```python
from build123d import *

# Parameters (mm, degrees)
F0_R     = 21.5
F1_DEPTH = 3
F2_R     = 1
F3_DEPTH = 3
F4_D     = 3


with BuildPart() as f1:
    # F0 (on Top) → F1 (new body)
    with BuildSketch(Plane.XY):
        Circle(F0_R)
    extrude(amount=F1_DEPTH)

    # F2 (on face) → F3 (join)
    with BuildSketch(Plane.XY.offset(3)):
        with BuildLine():
            Line((-1.347391, 11.193886), (0, 21.5))
            Line((0, 21.5), (-4.736634, 11.324242))
            Line((-4.736634, 11.324242), (-1.543514, 3.690199))
            ThreePointArc((-1.543514, 3.690199), (-3.859717, 1.050041), (-3.200264, -2.399647))
            Line((-3.200264, -2.399647), (-9.020494, -6.763818))
            Line((-9.020494, -6.763818), (-18.619546, -10.75))
            Line((-18.619546, -10.75), (-7.438764, -9.764166))
            Line((-7.438764, -9.764166), (-2.424049, -3.181821))
            ThreePointArc((-2.424049, -3.181821), (1.020496, -3.867633), (3.678288, -1.571687))
            Line((3.678288, -1.571687), (10.367886, -4.430068))
            Line((10.367886, -4.430068), (18.619546, -10.75))
            Line((18.619546, -10.75), (12.175398, -1.560076))
            Line((12.175398, -1.560076), (3.967563, -0.508377))
            ThreePointArc((3.967563, -0.508377), (2.839221, 2.817592), (-0.478023, 3.971334))
            Line((-0.478023, 3.971334), (-1.347391, 11.193886))
        make_face()
        Circle(F2_R, mode=Mode.SUBTRACT)
    extrude(amount=F3_DEPTH)

    # F4 (through all)
    with Locations(Plane(origin=(0, 0, 0), x_dir=(1, 0, 0), z_dir=(0, 0, -1))):
        with Locations((0, 0)):
            Hole(F4_D / 2)


solid = f1.part
```
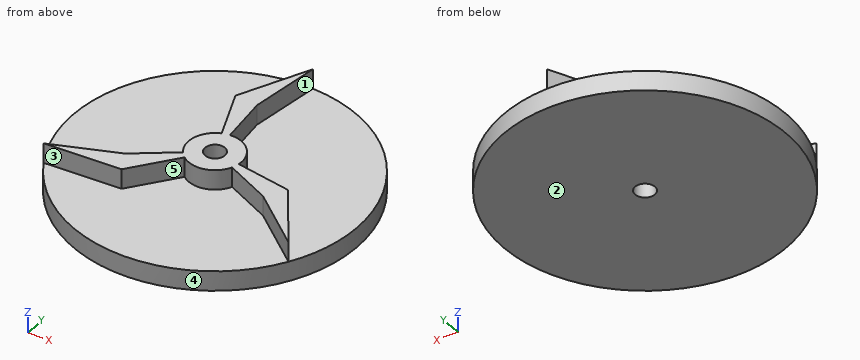
For this review, take the finished solid that the model builds, in its own axes (mm). Face numbers are marked on the shaded views. A direction names the side the tool comes from. Give positions to 0.01 mm unless a question says otherwise; leave off trailing zeros. Write each loop counter-clockwise with the first axis right and the second up, starting at its lowest first coordinate (ties: lowest second). Pieces come first, ordered by that corner, then holes. Notation, with made-up numbers: M 10,81 L 21,81 A32 cw 21,110 Z; hole C 65.5,35.5 d1. An arc over 180 degrees is marked long. One line per item, written item: value.
1) Take a section at D-D, the plane y = -8. Write out the cut boundary in (x, z).
Results are:
outline: M -19.96,0 L 19.96,0 L 19.96,3 L 16.69,3 L 16.69,6 L 15.03,6 L 15.03,3 L -6.09,3 L -6.09,6 L -12,6 L -12,3 L -19.96,3 Z
2) Take a section at A-A, the plane y = 0. Write out the cut boundary in (x, z), then the cut area to 3 significant figures.
Results are:
outline: M -21.5,0 L -1.5,0 L -1.5,6 L -4,6 L -4,3 L -21.5,3 Z; M 1.5,0 L 21.5,0 L 21.5,3 L 4,3 L 4,6 L 1.5,6 Z
area: 135 mm²
3) For line 1 (Y direction, x = 0, z = 1.35); line 2 (Z direction, x = 16, y = -4); line 3 (Y direction, x = -3.5, z = 4.85), list the stretches that pass through material, from the lowest coordinate up. Write a range as from..to.
Results are:
line 1: y = -21.5..-1.5, 1.5..21.5
line 2: z = 0..3
line 3: y = -4.59..-2.62, -1.94..1.94, 8.37..13.98
4) For P1, Ø1, axis at y = 6.5, z = 2, coming from the -X side; P2, Ø11, axis at x = -13, y = 13, coming from the +Z side; P3, Ø1.5, axis at x = -10.5, z = 3, coming from the -Y side, all flat-tipped, find the tip position at first contact; note any pin that passes through.
Results are:
P1: stops at x = -20.65
P2: stops at z = 3
P3: stops at y = -19.16
5) Take a section at C-C, the plane x = 18. Write out the cut boundary in (y, z), then the cut area to 3 significant figures.
Results are:
outline: M -11.76,0 L 11.76,0 L 11.76,3 L -9.87,3 L -9.87,6 L -10.28,6 L -10.28,3 L -11.76,3 Z
area: 71.8 mm²
6) The part is to be moulded in two halves that separate along X. For the marked faces 1, 2 and 3, say which applies: +X half, -X half, draft (parallel to the pull), parting line (faces both ways), or undercut.
Results are:
face 1: +X half
face 2: draft
face 3: undercut
7) For the marked faces 4 and 5, list the 3-axis set-ups (+Z, -Z, +X, -X, +Y, -Y) from which the entire face can be reached by the end or side of a thin tool; tool diameter is ignored.
Results are:
face 4: +Z, -Z
face 5: +Z, -Y
8) Take a section at B-B, the plane z = 5.4. Write out the cut boundary in (x, y).
Results are:
outline: M -18.62,-10.75 L -7.44,-9.76 L -2.42,-3.18 A4 ccw 3.68,-1.57 L 10.37,-4.43 L 18.62,-10.75 L 12.18,-1.56 L 3.97,-0.51 A4 ccw -0.48,3.97 L -1.35,11.19 L 0,21.5 L -4.74,11.32 L -1.54,3.69 A4 ccw -3.2,-2.4 L -9.02,-6.76 Z; hole C 0,0 d3
